from build123d import *

# Parameters (mm, degrees)
SKETCH4_W           = 35
SKETCH4_H           = 35
BOSS_EXTRUDE2_DEPTH = 48.050661441
SKETCH5_R           = 7.5
CUT_EXTRUDE1_DEPTH  = 44


with BuildPart() as part:
    # Sweep1: sweep along a path in Sketch3
    with BuildLine(Plane(origin=(0, 0, 0), x_dir=(1, 0, 0), z_dir=(0, 1, 0))) as sweep1_path:
        Line((55.06330006, -48.050661441), (46.590672007, 0))
    # Sketch1<2> → Sweep1 (sweep)
    with BuildSketch(Plane.XY):
        Polygon((0, 25), (0, -25), (15, -25), (15, -15), (35, -15), (35, -35), (-10, -35), (-10, 35), (35, 35), (35, 15), (15, 15), (15, 25), align=None)
    sweep(path=sweep1_path.line)

    # Sketch4 → Boss-Extrude2 (add)
    with BuildSketch(Plane.XY):
        with Locations((-17.5, 17.5)):
            Rectangle(SKETCH4_W, SKETCH4_H)
    extrude(amount=BOSS_EXTRUDE2_DEPTH)

    # Sketch5 → Cut-Extrude1 (cut)
    with BuildSketch(Plane(origin=(0, 35, 0), x_dir=(1, 0, 0), z_dir=(0, 1, 0))):
        with Locations(Location((-20, -25, 0), (0, 0, 270))):
            Circle(SKETCH5_R)
    extrude(amount=-CUT_EXTRUDE1_DEPTH, mode=Mode.SUBTRACT)


solid = part.part
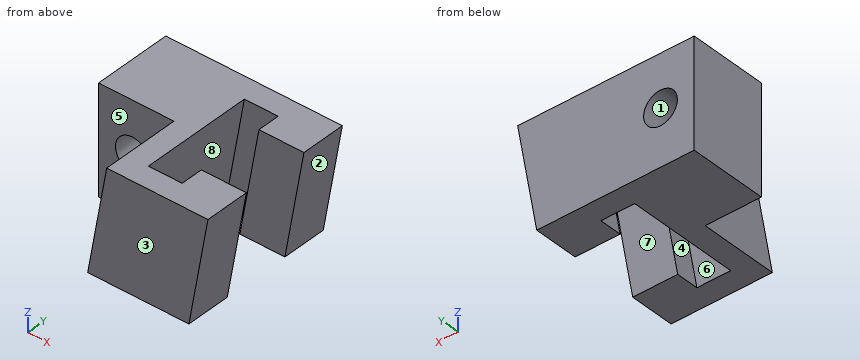
Design review of the part built by this model. Coordinates are the model's own, in mm. Face numbers are marked on the shaded views. A direction names the side the tool comes from. Round coordinates to 2 decimals unless told otherwise and drop trailing zeros. Write each loop counter-clockwise with the first axis right and the second up, starting at its lowest first coordinate (ties: lowest second). Pieces come first, ordered by that corner, then holes. Notation, with made-up numbers: (-2.5, -28) -> (45.5, -28) arc R22 cw to (45.5, 9) -> close; hole circle Ø6 at (85.5, 27). An arc over 180 degrees is marked (long way). One line per question, with ' | ' between items.
(1) Take a section at B-B, the plane y = 30.5. State the section outline as (x, z) points.
Result sheet:
outline: (-35, 0) -> (35, 0) -> (43.47, 48.05) -> (-35, 48.05) -> close; hole circle Ø15 at (-20, 25)
(2) Wall thickness on line 1 (X direction, y = 19, z = 25); line 2 (Y direction, x = -21, z = 3); line 3 (X direction, y = 18, z = 33): over which ranges is each line inside the solid? List them lowest first. Write a range as [from, to].
Result sheet:
line 1: [-35, -27.5], [-12.5, 4.41], [19.41, 39.41] | line 2: [0, 35] | line 3: [-35, 5.82], [20.82, 40.82]
(3) Take a section at A-A, the plane x = -20. State the section outline as (y, z) points.
Result sheet:
outline: (0, 0) -> (35, 0) -> (35, 17.5) -> (0, 17.5) -> close; (0, 32.5) -> (35, 32.5) -> (35, 48.05) -> (0, 48.05) -> close
(4) Take a section at C-C, the plane z = 20. State the section outline as (x, y) points, and give its area (3 significant figures).
Result sheet:
outline: (-35, 0) -> (-25.59, 0) -> (-25.59, 35) -> (-35, 35) -> close; (-14.41, 0) -> (-6.47, 0) -> (-6.47, -35) -> (38.53, -35) -> (38.53, -15) -> (18.53, -15) -> (18.53, -25) -> (3.53, -25) -> (3.53, 25) -> (18.53, 25) -> (18.53, 15) -> (38.53, 15) -> (38.53, 35) -> (-14.41, 35) -> close | area: 2,410 mm2
(5) Insertion check: P1, Ø12, axis at x = -20.5, z = 29, coming from the -Y side; P2, Ø1, axis at y = -21.5, z = 41.5, coming from the -X side; P3, Ø9, axis at x = -20, z = 25, coming from the +Y side; P4, Ø4, axis at y = 25, z = 23.5, coming from the +X side. Each pin has a flat end and moves straight along its axis. Give the tip position at first contact, or say it passes through.
Result sheet:
P1: y = 0 | P2: x = -2.77 | P3: through | P4: x = 39.5
(6) Machinability: for the marked faces 4, 5, 6, 7 and 8, which of the approach directions +Z, -Z, +X, -X, +Y, -Y give a long, thin tool a straight path to every point of the face, cutting with its end or side? Answer none if there is none.
Result sheet:
face 4: +Z | face 5: +Z, -X, -Y | face 6: none | face 7: +Z, -Z, +X | face 8: -Z
(7) Take a section at D-D, the plane z = 38.5. State the section outline as (x, y) points.
Result sheet:
outline: (-35, 0) -> (-3.21, 0) -> (-3.21, -35) -> (41.79, -35) -> (41.79, -15) -> (21.79, -15) -> (21.79, -25) -> (6.79, -25) -> (6.79, 25) -> (21.79, 25) -> (21.79, 15) -> (41.79, 15) -> (41.79, 35) -> (-35, 35) -> close
(8) Draft analysis for pull direction X (two halves, no side actions). For the marked faces 1, 2 and 3, state which applies: released by +X, released by -X, zero draft, split by the parting line, or undercut.
Result sheet:
face 1: undercut | face 2: released by +X | face 3: zero draft
